Geometry check sheet. Reference: the model listing, model coordinates, mm. A direction names the side the tool comes from. Coordinates: 2 decimals unless noted, no trailing zeros. Loops run counter-clockwise (first coordinate to the right, second up) from the corner with the lowest first, then second, coordinate; pieces in that order, holes last.
from build123d import *

# Parameters (mm, degrees)
F0_W     = 27.3
F0_H     = 27.3
F0_R     = 1.5
F1_DEPTH = 2
F2_SIZE  = 2
F3_W     = 27.3
F3_H     = 15
F4_DEPTH = 3
F5_R     = 1


with BuildPart() as f1:
    # F0 (on Top) → F1 (new body)
    with BuildSketch(Plane.XY):
        with Locations((-0.626242, 1.435703)):
            Rectangle(F0_W, F0_H)
        with Locations((-10.890681, -9.214297)):
            Circle(F0_R, mode=Mode.SUBTRACT)
        with Locations((9.809319, -9.214297)):
            Circle(F0_R, mode=Mode.SUBTRACT)
        with Locations((-10.890681, 12.085703)):
            Circle(F0_R, mode=Mode.SUBTRACT)
        with Locations((9.809319, 12.085703)):
            Circle(F0_R, mode=Mode.SUBTRACT)
    extrude(amount=F1_DEPTH)

    # F2
    f2_edges = [f1.edges().sort_by_distance(p)[0] for p in [
        (13.023758, 15.085703, 1),
        (13.023758, -12.214297, 1),
        (-14.276242, -12.214297, 1),
        (-14.276242, 15.085703, 1),
    ]]
    chamfer(f2_edges, length=F2_SIZE)

    # F3 (on face) → F4 (join)
    with BuildSketch(Plane.XY.offset(2)):
        with Locations((-0.626242, 2.082483)):
            Rectangle(F3_W, F3_H)
    extrude(amount=F4_DEPTH)

    # F5
    f5_edges = [f1.edges().sort_by_distance(p)[0] for p in [
        (-0.626242, 9.582483, 5),
        (-0.626242, -5.417517, 5),
        (-14.276242, 2.082483, 5),
        (13.023758, 2.082483, 5),
    ]]
    fillet(f5_edges, radius=F5_R)


solid = f1.part
1) Material ranges on probe 1 along X at (y, z) = (12, 0.9); probe 2 along X at (y, z) = (10.75, 1.1); probe 3 along Y at (x, z) = (-12, 1.4), recorded low to high.
Data:
probe 1: x = -14.28 to -12.39, -9.39 to 8.31, 11.31 to 13.02
probe 2: x = -14.28 to -11.57, -10.21 to 9.13, 10.49 to 13.02
probe 3: y = -12.21 to -10.22, -8.2 to 11.08, 13.1 to 15.09
2) Section check D-D on z = 2.5. Record the cut outline in (x, y).
Data:
outline: (-14.28, -5.42) - (13.02, -5.42) - (13.02, 9.58) - (-14.28, 9.58) - close
3) Access from +Z, -Z, +X, -X, +Y, -Y to the whole of each face (thin tool, end or side, straight path). Record for faces 4 (the flat face through (-1, 12, 2)), 5 (the flat face through (-1, -5.418, 3)), 6 (the flat face through (12.04, -11.2, 0.99)).
Data:
face 4: +Z, +X, -X, +Y
face 5: +Z, +X, -X, -Y
face 6: +Z, -Z, +X, -Y
4) Section check C-C on x = -9.75. Record the cut outline in (y, z).
Data:
outline: (-12.21, 0) - (-10.19, 0) - (-10.19, 2) - (-12.21, 2) - close; (-8.24, 0) - (11.11, 0) - (11.11, 2) - (9.58, 2) - (9.58, 4) arc R1 ccw to (8.58, 5) - (-4.42, 5) arc R1 ccw to (-5.42, 4) - (-5.42, 2) - (-8.24, 2) - close; (13.06, 0) - (15.09, 0) - (15.09, 2) - (13.06, 2) - close
5) Mould release check, pull along Y, two halves, no side actions. Record for faces 1 (the flat face through (-1, 2, 0)), 2 (the cylindrical face through (10.501, 10.755, 0.986)), 3 (the flat face through (-13.26, 14.1, 0.99)): +Y half, -Y half, draft (parallel to the pull), parting line (faces both ways), or undercut.
Data:
face 1: draft
face 2: undercut
face 3: +Y half
6) Depth check by flat-ended pin: pin 1 (2 mm diameter, centred on x = 5.5, z = 3.5, fed in from +Y); pin 2 (2.5 mm diameter, centred on x = 9.81, y = 12.09, fed in from +Z); pin 3 (4 mm diameter, centred on x = -10.89, y = -9.21, fed in from +Z). Enter the tip coordinate at first touch or a pass-through.
Data:
pin 1: stops at y = 9.58
pin 2: passes through
pin 3: stops at z = 2
7) Section check B-B on z = 0.85. Record the cut outline in (x, y), and give its area (3 significant figures).
Data:
outline: (-14.28, -10.21) - (-12.28, -12.21) - (11.02, -12.21) - (13.02, -10.21) - (13.02, 13.09) - (11.02, 15.09) - (-12.28, 15.09) - (-14.28, 13.09) - close; hole circle Ø3 at (-10.89, -9.21); hole circle Ø3 at (-10.89, 12.09); hole circle Ø3 at (9.81, -9.21); hole circle Ø3 at (9.81, 12.09)
area: 709 mm2
8) Section check A-A on x = 5. Record the cut outline in (y, z), and give its area (3 significant figures).
Data:
outline: (-12.21, 0) - (15.09, 0) - (15.09, 2) - (9.58, 2) - (9.58, 4) arc R1 ccw to (8.58, 5) - (-4.42, 5) arc R1 ccw to (-5.42, 4) - (-5.42, 2) - (-12.21, 2) - close
area: 99.2 mm2
